The listing builds one solid part. Answer for the finished solid, in the listing's coordinates (mm). Round coordinates to 2 decimals unless told otherwise and drop trailing zeros. Write each loop counter-clockwise with the first axis right and the second up, starting at its lowest first coordinate (ties: lowest second). Pieces come first, ordered by that corner, then holes.
Item 1: Each of these flat-tipped pins is pushed along its axis until it touches: pin 1 (8 mm diameter, centred on y = 72.5, z = -16.5, fed in from -X); pin 2 (10 mm diameter, centred on y = 116, z = -4.5, fed in from -X); pin 3 (15 mm diameter, centred on x = -15, z = -1, fed in from +Y); pin 4 (2 mm diameter, centred on y = 153, z = 13, fed in from +X). Where does it stop, or does it pass through?
Item 2: Find section A-A on x = 0. Give the vertices of the cut face in (y, z).
Item 3: Find section C-C on x = -19. Give the vertices of the cut face in (y, z).
Item 4: Find the intervals of material crossed by probe 1 along X at (y, z) = (30.5, -1); probe 2 along X at (y, z) = (27, 18.5); probe 3 along X at (y, z) = (40, 0), in increasing order.
Item 5: Find section B-B on z = -3. Give the vertices of the cut face in (x, y).
Item 6: For a pull along Y with two mould halves and no side action, classify faces 1 (the face through (-23.3, 133, -0.1)), 2 (the face through (24.787, 84.796, -3.255)), 3 (the face through (-22.1, 172, 7.3)) as +Y half, -Y half, draft (parallel to the pull), parting line (faces both ways), or undercut.
Item 7: Find section D-D on y = 153. Give the vertices of the cut face in (x, z).
```python
from build123d import *

# Parameters (mm, degrees)
SKETCH_1_R          = 25
SKETCH_1_R_2        = 23
EXTRUDE_1_DEPTH     = 172
CUT_EXTRUDE_1_DEPTH = 102


with BuildPart() as part:
    # Эскиз1 → Бобышка-Вытянуть1 (new body)
    with BuildSketch(Plane(origin=(0, 0, 0), x_dir=(1, 0, 0), z_dir=(0, 1, 0))):
        with Locations(Location((0, 0, 0), (0, 0, 270))):
            Circle(SKETCH_1_R)
        with Locations(Location((0, 0, 0), (0, 0, 270))):
            Circle(SKETCH_1_R_2, mode=Mode.SUBTRACT)
    extrude(amount=EXTRUDE_1_DEPTH)

    # Эскиз2 → Вырез-Вытянуть1 (cut)
    with BuildSketch(Plane(origin=(0, 31, 0), x_dir=(-1, 0, 0), z_dir=(0, -1, 0))):
        Polygon((0, 0), (29.61457633, 51.293950849), (33.452789958, -57.941931861), align=None)
    extrude(amount=-CUT_EXTRUDE_1_DEPTH, mode=Mode.SUBTRACT)


solid = part.part
```
Check values:
1. pin 1: stops at x = -11.84
1. pin 2: stops at x = 20.95
1. pin 3: passes through
1. pin 4: stops at x = 21.93
2. outline: (0, -25) - (172, -25) - (172, -23) - (0, -23) - close; (0, 23) - (172, 23) - (172, 25) - (0, 25) - close
3. outline: (0, -16.25) - (31, -16.25) - (31, -12.96) - (0, -12.96) - close; (0, 12.96) - (31, 12.96) - (31, 16.25) - (0, 16.25) - close; (133, -16.25) - (172, -16.25) - (172, -12.96) - (133, -12.96) - close; (133, 12.96) - (172, 12.96) - (172, 16.25) - (133, 16.25) - close
4. probe 1: x = -24.98 to -22.98, 22.98 to 24.98
4. probe 2: x = -16.82 to -13.67, 13.67 to 16.82
4. probe 3: x = 23 to 25
5. outline: (-24.82, 0) - (-22.8, 0) - (-22.8, 31) - (-24.82, 31) - close; (-24.82, 133) - (-22.8, 133) - (-22.8, 172) - (-24.82, 172) - close; (22.8, 0) - (24.82, 0) - (24.82, 172) - (22.8, 172) - close
6. face 1: undercut
6. face 2: draft
6. face 3: +Y half
7. outline: circle Ø50 at (0, 0); hole circle Ø46 at (0, 0)
